Here's how the part is built. I have some questions about the finished solid (model axes, mm). A direction names the side the tool comes from. Round coordinates to 2 decimals unless told otherwise and drop trailing zeros. Write each loop counter-clockwise with the first axis right and the second up, starting at its lowest first coordinate (ties: lowest second). Pieces come first, ordered by that corner, then holes. Notation, with made-up numbers: (42.25, -21.75) -> (50.25, -21.75) arc R3 ccw to (50.25, -16.75) -> close; hole circle Ø8 at (88.5, 63.5). An arc over 180 degrees is marked (long way). Put each result on its own line as item: value. Start each with the question number.
1. Suppose I cut it at B-B (y = -1). Please give me the cut outline in (x, z), then the cut area to 3 significant figures.
2. For pin 1 (3 mm diameter, centred on y = 2.5, z = -8, fed in from +X); pin 2 (2 mm diameter, centred on y = -0.5, z = -8, fed in from -X), each with a flat end and sliding along its axis, tell me the tip position at first contact or that it passes through.
3. Which directions (+Z, -Z, +X, -X, +Y, -Y) give clear straight access to the entire face, cutting with the end or side of a thin tool? Please do faces 1 (the face through (3.48, 1.97, 1.73)), 2 (the face through (2, 2, 0)).
4. Suppose I cut it at C-C (z = -4). Please give me the cut outline in (x, y), then the cut area to 3 significant figures.
5. We'd pull the mould along X, two halves only. Please class faces 3 (the face through (-3.48, -1.97, 1.73)), 4 (the face through (-2.5, -0.1, -9.9)), 5 (the face through (3.448, -2.028, 1.726)), 6 (the face through (0, 4, 2)): +X half, -X half, draft (parallel to the pull), parting line (faces both ways), or undercut.
6. I need wall thicknesses on probe 1 along Y at (x, z) = (0, -1.25); probe 2 along Z at (x, y) = (-1.5, 3); probe 3 along X at (y, z) = (2.25, -3). Which ranges of each line are inside material? Lowest first, please. Write a range as from..to.
7. Suppose I cut it at D-D (x = -4). Please give me the cut outline in (y, z), then the cut area to 3 significant figures.
8. Suppose I cut it at A-A (x = -1.5). Please give me the cut outline in (y, z).
```python
from build123d import *

# Parameters (mm, degrees)
SALIENTE_EXTRUIR1_DEPTH = 3.5
CROQUIS2_R              = 2.5
SALIENTE_EXTRUIR2_DEPTH = 20


with BuildPart() as part:
    # Croquis1 → Saliente-Extruir1 (new body)
    with BuildSketch(Plane.XY):
        Polygon((4.618802154, 0), (2.309401077, 4), (-2.309401077, 4), (-4.618802154, 0), (-2.309401077, -4), (2.309401077, -4), align=None)
    extrude(amount=SALIENTE_EXTRUIR1_DEPTH)

    # Croquis2 → Saliente-Extruir2 (add)
    with BuildSketch(Plane(origin=(0, 0, 0), x_dir=(-1, 0, 0), z_dir=(0, 0, -1))):
        with Locations(Location((0, 0, 0), (0, 0, 180))):
            Circle(CROQUIS2_R)
    extrude(amount=SALIENTE_EXTRUIR2_DEPTH)


solid = part.part
```
Verdict:
1. outline: (-4.04, 0) -> (-2.29, 0) -> (-2.29, -20) -> (2.29, -20) -> (2.29, 0) -> (4.04, 0) -> (4.04, 3.5) -> (-4.04, 3.5) -> close
1. area: 120 mm^2
2. pin 1: stops at x = 2.29
2. pin 2: stops at x = -2.5
3. face 1: +Z, -Z, +X, +Y
3. face 2: -Z
4. outline: circle Ø5 at (0, 0)
4. area: 19.6 mm^2
5. face 3: -X half
5. face 4: parting line
5. face 5: +X half
5. face 6: draft
6. probe 1: y = -2.5..2.5
6. probe 2: z = 0..3.5
6. probe 3: x = -1.09..1.09
7. outline: (-1.07, 0) -> (1.07, 0) -> (1.07, 3.5) -> (-1.07, 3.5) -> close
7. area: 7.50 mm^2
8. outline: (-4, 0) -> (-2, 0) -> (-2, -20) -> (2, -20) -> (2, 0) -> (4, 0) -> (4, 3.5) -> (-4, 3.5) -> close
